from build123d import *

# Parameters (mm, degrees)
F0_R     = 2.75
F0_R_2   = 20
F1_DEPTH = 10


with BuildPart() as f1:
    # F0 (on Top) → F1 (new body)
    with BuildSketch(Plane.XY):
        with BuildLine():
            Line((-50, -60), (50, -60))
            ThreePointArc((50, -60), (57.071068, -57.071068), (60, -50))
            Line((60, -50), (60, 50))
            ThreePointArc((60, 50), (57.071068, 57.071068), (50, 60))
            Line((50, 60), (-50, 60))
            ThreePointArc((-50, 60), (-57.071068, 57.071068), (-60, 50))
            Line((-60, 50), (-60, -50))
            ThreePointArc((-60, -50), (-57.071068, -57.071068), (-50, -60))
        make_face()
        with Locations((-46, -46)):
            Circle(F0_R, mode=Mode.SUBTRACT)
        with BuildLine():
            Line((-33.480436, 22.550578), (-33.480436, -22.449422))
            ThreePointArc((-33.480436, -22.449422), (-40.929516, -30.050748), (-48.480436, -22.550578))
            Line((-48.480436, -22.550578), (-48.480436, 22.449422))
            ThreePointArc((-48.480436, 22.449422), (-41.030674, 29.949593), (-33.480436, 22.550578))
        make_face(mode=Mode.SUBTRACT)
        with Locations((-18.384776, -18.384776)):
            Circle(F0_R, mode=Mode.SUBTRACT)
        with BuildLine():
            Line((-22.550578, -33.480436), (22.449422, -33.480436))
            ThreePointArc((22.449422, -33.480436), (29.949593, -40.930199), (22.550578, -48.480436))
            Line((22.550578, -48.480436), (-22.449422, -48.480436))
            ThreePointArc((-22.449422, -48.480436), (-29.949593, -41.030674), (-22.550578, -33.480436))
        make_face(mode=Mode.SUBTRACT)
        with Locations((46, -46)):
            Circle(F0_R, mode=Mode.SUBTRACT)
        with Locations((18.384776, -18.384776)):
            Circle(F0_R, mode=Mode.SUBTRACT)
        with Locations((-18.384776, 18.384776)):
            Circle(F0_R, mode=Mode.SUBTRACT)
        with Locations((-46, 46)):
            Circle(F0_R, mode=Mode.SUBTRACT)
        Circle(F0_R_2, mode=Mode.SUBTRACT)
        with Locations((18.384776, 18.384776)):
            Circle(F0_R, mode=Mode.SUBTRACT)
        with BuildLine():
            Line((48.480436, 22.449422), (48.480436, -22.550578))
            ThreePointArc((48.480436, -22.550578), (40.930199, -29.949593), (33.480436, -22.449422))
            Line((33.480436, -22.449422), (33.480436, 22.550578))
            ThreePointArc((33.480436, 22.550578), (41.031356, 30.050748), (48.480436, 22.449422))
        make_face(mode=Mode.SUBTRACT)
        with BuildLine():
            ThreePointArc((22.550578, 48.480436), (30.050748, 40.929516), (22.449422, 33.480436))
            Line((22.449422, 33.480436), (-22.550578, 33.480436))
            ThreePointArc((-22.550578, 33.480436), (-29.949593, 41.030674), (-22.449422, 48.480436))
            Line((-22.449422, 48.480436), (22.550578, 48.480436))
        make_face(mode=Mode.SUBTRACT)
        with Locations((46, 46)):
            Circle(F0_R, mode=Mode.SUBTRACT)
    extrude(amount=F1_DEPTH)


solid = f1.part
Check sheet for the modelled part. Datum: model origin and axes. Units: mm. A direction names the side the tool comes from. Coordinates: 2 decimals unless noted, no trailing zeros. Write each loop counter-clockwise with the first axis right and the second up, starting at its lowest first coordinate (ties: lowest second). Pieces come first, ordered by that corner, then holes.
Item 1: Cross-section at A-A on x = 0. Record the boundary of the cut face in (y, z).
Numbers:
outline: (-60, 0) - (-48.48, 0) - (-48.48, 10) - (-60, 10) - close; (-33.48, 0) - (-20, 0) - (-20, 10) - (-33.48, 10) - close; (20, 0) - (33.48, 0) - (33.48, 10) - (20, 10) - close; (48.48, 0) - (60, 0) - (60, 10) - (48.48, 10) - close
Item 2: Cross-section at C-C on x = 38.5. Record the boundary of the cut face in (y, z), then the cut area to 3 significant figures.
Numbers:
outline: (-60, 0) - (-29.53, 0) - (-29.53, 10) - (-60, 10) - close; (29.63, 0) - (60, 0) - (60, 10) - (29.63, 10) - close
area: 608 mm2
Item 3: Scan lines: probe 1 along Y at (x, z) = (-1, 7.75); probe 2 along Y at (x, z) = (7.5, 1.5); probe 3 along X at (y, z) = (-41.5, 3.75). Record each from-to range of solid material in increasing order.
Numbers:
probe 1: y = -60 to -48.48, -33.48 to -19.97, 19.97 to 33.48, 48.48 to 60
probe 2: y = -60 to -48.48, -33.48 to -18.54, 18.54 to 33.48, 48.48 to 60
probe 3: x = -60 to -29.93, 29.93 to 60
Item 4: Access from +Z, -Z, +X, -X, +Y, -Y to the whole of each face (thin tool, end or side, straight path). Record for faces 4 (the face through (0, -33.48, 5)), 5 (the face through (1, 60, 5)).
Numbers:
face 4: +Z, -Z
face 5: +Z, -Z, +X, -X, +Y
Item 5: Mould release check, pull along X, two halves, no side actions. Record for faces 1 (the face through (-29.95, 40.87, 4.93)), 2 (the face through (-60, 1, 5)), 3 (the face through (-28, 1, 0)): released by +X, released by -X, zero draft, split by the parting line, or undercut.
Numbers:
face 1: undercut
face 2: released by -X
face 3: zero draft
Item 6: Cross-section at D-D on y = 39. Record the boundary of the cut face in (x, z), then the cut area to 3 significant figures.
Numbers:
outline: (-60, 0) - (-29.68, 0) - (-29.68, 10) - (-60, 10) - close; (29.78, 0) - (60, 0) - (60, 10) - (29.78, 10) - close
area: 605 mm2
